Verification items for this drawing (mm, ordinates from the low corner). A direction names the side the tool comes from. Give positions to 0.01 mm unless a question says otherwise; leave off trailing zeros. Write each loop counter-clockwise with the first axis right and the second up, starting at its lowest first coordinate (ties: lowest second). Pieces come first, ordered by that corner, then holes. Notation, with made-up numbers: M 3.5,31.5 L 45.5,31.5 A25 ccw 45.5,45.5 Z; hole C -1.5,-38.75 d6. An arc over 180 degrees is marked long. Use one line per item in the form item = value. Start each with the question number.
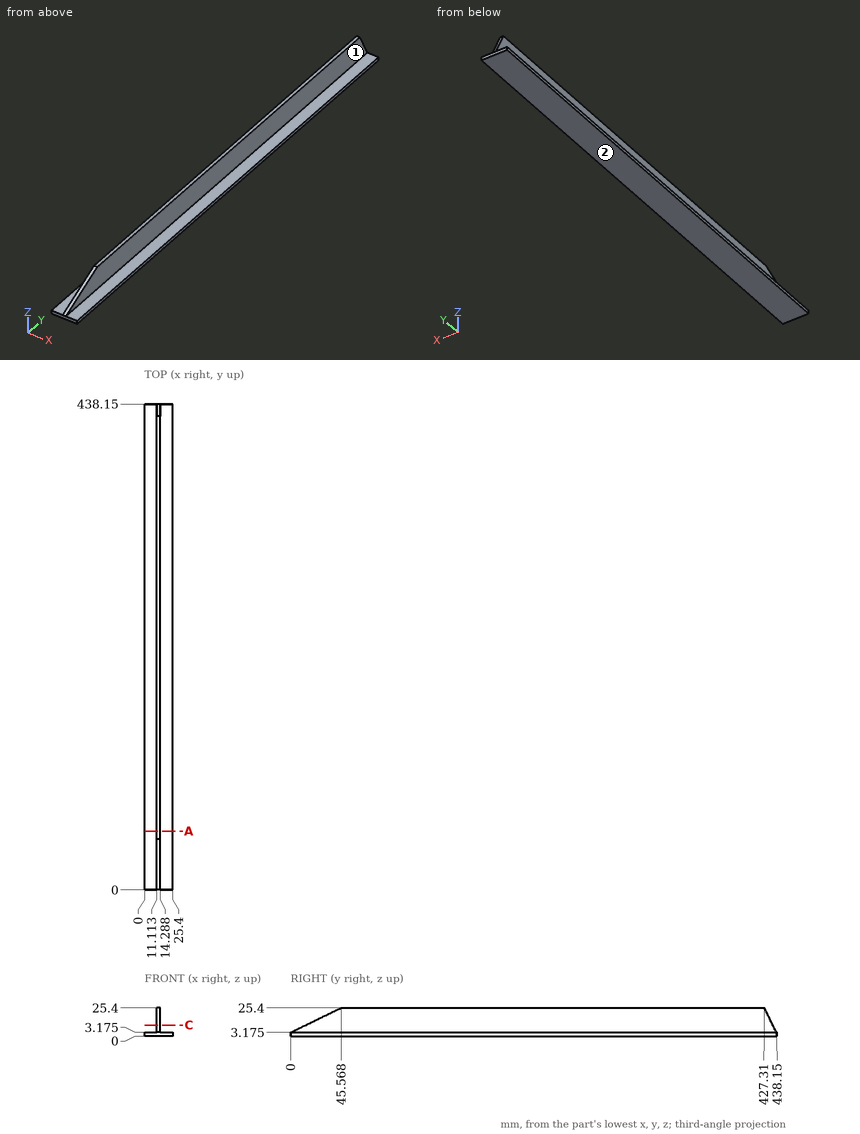
(1) Thickness scan on probe 1 along Z at (x, y) = (17.25, 195) (1 decimal); probe 2 along X at (y, z) = (304, 12.5); probe 3 along Y at (x, z) = (11.25, 7) (1 decimal). Record the ranges inside material, lowest first. Write a range as [from, to].
(2) Tool access check on the marked faces 1 and 2. Record the directions out of +Z, -Z, +X, -X, +Y, -Y that give a thin tool (end or side, any length) a straight path to the whole face; none if there is none.
(3) Sectioned sample at C-C, the plane z = 9.75. Record the boundary of the cut face in (x, y), plus the area to 3 significant figures.
(4) Sectioned sample at A-A, the plane y = 53. Record the boundary of the cut face in (x, z) (1 decimal).
(5) Depth check by flat-ended pin: pin 1 (1 mm diameter, centred on y = 78, z = 5.5, fed in from -X); pin 2 (9 mm diameter, centred on x = 20, y = 192.5, fed in from +Z) (1 decimal); pin 3 (8 mm diameter, centred on x = 21, z = 14.5, fed in from -Y); pin 4 (1.5 mm diameter, centred on y = 166, z = 20.5, fed in from +X). Enter the tip coordinate at first touch or a pass-through.
Numbers:
q1.probe_1 = [0, 3.2]
q1.probe_2 = [11.11, 14.29]
q1.probe_3 = [7.8, 436.3]
q2.face_1 = +Z, +X, +Y, -Y
q2.face_2 = -Z, +X, -X, +Y, -Y
q3.outline = M 11.11,13.48 L 14.29,13.48 L 14.29,434.94 L 11.11,434.94 Z
q3.area = 1,340 mm2
q4.outline = M 0,0 L 25.4,0 L 25.4,3.2 L 14.3,3.2 L 14.3,25.4 L 11.1,25.4 L 11.1,3.2 L 0,3.2 Z
q5.pin_1 = 11.11
q5.pin_2 = 3.2
q5.pin_3 = through
q5.pin_4 = 14.29
